from build123d import *

# Parameters (mm, degrees)
SKETCH1_W          = 35
SKETCH1_H          = 2.5
CUT_EXTRUDE1_START = -8
CUT_EXTRUDE1_DEPTH = 8
CUT_EXTRUDE2_DEPTH = 8
CHAMFER1_SIZE      = 0.5


with BuildPart() as part:
    # Sketch1 → Revolve1 (revolve)
    with BuildSketch(Plane(origin=(0, 0, 0), x_dir=(1, 0, 0), z_dir=(0, 1, 0))):
        with Locations((-17.5, 1.25)):
            Rectangle(SKETCH1_W, SKETCH1_H)
    revolve(axis=Axis((0, 0, 0), (-1, 0, 0)))

    # Sketch2 → Cut-Extrude1 (cut)
    with BuildSketch(Plane.ZY.offset(35).offset(CUT_EXTRUDE1_START)):
        with BuildLine():
            Line((-2, 1.5), (-2, -1.5))
            ThreePointArc((-2, -1.5), (-2.5, 0), (-2, 1.5))
        make_face()
    extrude(amount=CUT_EXTRUDE1_DEPTH, mode=Mode.SUBTRACT)

    # Sketch3 → Cut-Extrude2 (cut)
    with BuildSketch(Plane(origin=(0, 0, 0), x_dir=(0, 0, -1), z_dir=(1, 0, 0))):
        with BuildLine():
            Line((2, 1.5), (2, -1.5))
            ThreePointArc((2, -1.5), (2.5, 0), (2, 1.5))
        make_face()
    extrude(amount=-CUT_EXTRUDE2_DEPTH, mode=Mode.SUBTRACT)

    # Chamfer1
    chamfer1_edges = [part.edges().sort_by_distance(p)[0] for p in [
        (0, 0, 2.5),
        (-35, 0, 2.5),
    ]]
    chamfer(chamfer1_edges, length=CHAMFER1_SIZE - 0.0001)  # a hair under: the kernel refuses the full size


solid = part.part
Design review of the part built by this model. Coordinates are the model's own, in mm. A direction names the side the tool comes from. Coordinates: 2 decimals unless noted, no trailing zeros. Loops run counter-clockwise (first coordinate to the right, second up) from the corner with the lowest first, then second, coordinate; pieces in that order, holes last. Notation, with made-up numbers: M -9.75,84 L 49.25,84 A32 cw 49.25,119 Z; hole C 6,7 d3. An arc over 180 degrees is marked long. Use one line per item in the form item = value.
(1) Consider section A-A (x = -23.5). Write out the cut boundary in (y, z), and give its area (3 significant figures).
Return value:
outline = C 0,0 d5
area = 19.6 mm2
(2) Clearance check with flat-ended pins moving along their axes: P1, Ø1.5, axis at x = -20, z = -1, coming from the -Y side; P2, Ø2.5, axis at x = -2, y = 0, coming from the -Z side; P3, Ø1, axis at x = -28, y = -1.5, coming from the +Z side. State where each tip first meets the part, or that it passes through.
Return value:
P1 = -2.49
P2 = -2
P3 = 2.29
(3) For faces 1 (the face through (-17.3, -0.1, 2.5)), 2 (the face through (-4, 0, -2)), 3 (the face through (-31, 0, -2)), list the 3-axis set-ups (+Z, -Z, +X, -X, +Y, -Y) from which the entire face can be reached by the end or side of a thin tool; tool diameter is ignored.
Return value:
face_1 = +X, -X
face_2 = -Z, +X, +Y, -Y
face_3 = -Z, -X, +Y, -Y
(4) Consider section B-B (x = -4). Write out the cut boundary in (y, z), and give its area (3 significant figures).
Return value:
outline = M -1.5,-2 L 1.5,-2 A2.5 ccw long Z
area = 18.6 mm2
(5) For line 1 along Z through (x, y) = (-15, -1.5); line 2 along Z through (x, y) = (-4.5, 0.05); line 3 along Y through (x, z) = (-24, 2), list the stretches that pass through material, from the lowest coordinate up. Write a range as from..to.
Return value:
line_1 = -2..2
line_2 = -2..2.5
line_3 = -1.5..1.5
